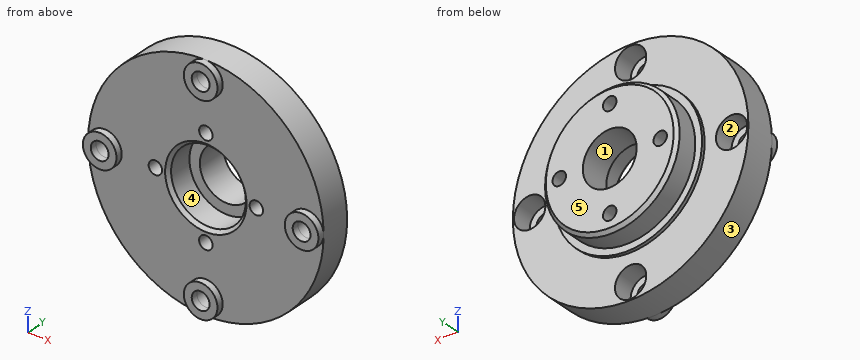
```python
from build123d import *

# Parameters (mm, degrees)
SKETCH1_R           = 35
SKETCH1_R_2         = 11.1
SKETCH1_R_3         = 2.65
BOSS_EXTRUDE1_DEPTH = 3
SKETCH2_R           = 35
SKETCH2_R_2         = 4.65
SKETCH2_R_3         = 11.1
BOSS_EXTRUDE2_DEPTH = 6
SKETCH3_R           = 11.1
SKETCH3_R_2         = 8
BOSS_EXTRUDE3_DEPTH = 1
SKETCH4_R           = 20
SKETCH4_R_2         = 8
BOSS_EXTRUDE4_DEPTH = 8
SKETCH5_R           = 22
SKETCH5_R_2         = 20
BOSS_EXTRUDE5_DEPTH = 1
SKETCH6_R           = 5
SKETCH6_R_2         = 2.65
BOSS_EXTRUDE6_DEPTH = 2
SKETCH7_R           = 2
CUT_EXTRUDE1_DEPTH  = 20
CHAMFER1_SIZE       = 1


with BuildPart() as part:
    # Sketch1 → Boss-Extrude1 (new body)
    with BuildSketch(Plane(origin=(0, 0, 0), x_dir=(1, 0, 0), z_dir=(0, 1, 0))):
        Circle(SKETCH1_R)
        Circle(SKETCH1_R_2, mode=Mode.SUBTRACT)
        with Locations((0, 30)):
            Circle(SKETCH1_R_3, mode=Mode.SUBTRACT)
        with Locations((30, 0)):
            Circle(SKETCH1_R_3, mode=Mode.SUBTRACT)
        with Locations((0, -30)):
            Circle(SKETCH1_R_3, mode=Mode.SUBTRACT)
        with Locations((-30, 0)):
            Circle(SKETCH1_R_3, mode=Mode.SUBTRACT)
    extrude(amount=BOSS_EXTRUDE1_DEPTH)

    # Sketch2 → Boss-Extrude2 (add)
    with BuildSketch(Plane(origin=(0, 3, 0), x_dir=(1, 0, 0), z_dir=(0, 1, 0))):
        Circle(SKETCH2_R)
        with Locations((0, -30)):
            Circle(SKETCH2_R_2, mode=Mode.SUBTRACT)
        with Locations((30, 0)):
            Circle(SKETCH2_R_2, mode=Mode.SUBTRACT)
        with Locations((0, 30)):
            Circle(SKETCH2_R_2, mode=Mode.SUBTRACT)
        with Locations((-30, 0)):
            Circle(SKETCH2_R_2, mode=Mode.SUBTRACT)
        Circle(SKETCH2_R_3, mode=Mode.SUBTRACT)
    extrude(amount=BOSS_EXTRUDE2_DEPTH)

    # Sketch3 → Boss-Extrude3 (add)
    with BuildSketch(Plane(origin=(0, 9, 0), x_dir=(1, 0, 0), z_dir=(0, 1, 0))):
        Circle(SKETCH3_R)
        Circle(SKETCH3_R_2, mode=Mode.SUBTRACT)
    extrude(amount=-BOSS_EXTRUDE3_DEPTH)

    # Sketch4 → Boss-Extrude4 (add)
    with BuildSketch(Plane(origin=(0, 9, 0), x_dir=(1, 0, 0), z_dir=(0, 1, 0))):
        Circle(SKETCH4_R)
        Circle(SKETCH4_R_2, mode=Mode.SUBTRACT)
    extrude(amount=BOSS_EXTRUDE4_DEPTH)

    # Sketch5 → Boss-Extrude5 (add)
    with BuildSketch(Plane(origin=(0, 9, 0), x_dir=(1, 0, 0), z_dir=(0, 1, 0))):
        Circle(SKETCH5_R)
        Circle(SKETCH5_R_2, mode=Mode.SUBTRACT)
    extrude(amount=BOSS_EXTRUDE5_DEPTH)

    # Sketch6 → Boss-Extrude6 (add)
    with BuildSketch(Plane(origin=(0, 0, 0), x_dir=(-1, 0, 0), z_dir=(0, -1, 0))):
        with Locations((30, 0)):
            Circle(SKETCH6_R)
        with Locations((30, 0)):
            Circle(SKETCH6_R_2, mode=Mode.SUBTRACT)
        with Locations((0, -30)):
            Circle(SKETCH6_R)
        with Locations((0, -30)):
            Circle(SKETCH6_R_2, mode=Mode.SUBTRACT)
        with Locations((-30, 0)):
            Circle(SKETCH6_R)
        with Locations((-30, 0)):
            Circle(SKETCH6_R_2, mode=Mode.SUBTRACT)
        with Locations((0, 30)):
            Circle(SKETCH6_R)
        with Locations((0, 30)):
            Circle(SKETCH6_R_2, mode=Mode.SUBTRACT)
    extrude(amount=BOSS_EXTRUDE6_DEPTH)

    # Sketch7 → Cut-Extrude1 (cut, through all)
    with BuildSketch(Plane(origin=(0, 17, 0), x_dir=(1, 0, 0), z_dir=(0, 1, 0))):
        with Locations((0, 15)):
            Circle(SKETCH7_R)
        with Locations((15, 0)):
            Circle(SKETCH7_R)
        with Locations((0, -15)):
            Circle(SKETCH7_R)
        with Locations((-15, 0)):
            Circle(SKETCH7_R)
    extrude(amount=-CUT_EXTRUDE1_DEPTH, mode=Mode.SUBTRACT)

    # Chamfer1
    chamfer1_edges = [part.edges().sort_by_distance(p)[0] for p in [
        (-11.1, 0, 0),
        (-20, 17, 0),
    ]]
    chamfer(chamfer1_edges, length=CHAMFER1_SIZE)


solid = part.part
```
Model file for the job. Use its own axes, mm. Face numbers are marked on the shaded views. A direction names the side the tool comes from. Coordinates: 2 decimals unless noted, no trailing zeros. Order: outer loops, then holes, each group sorted by start corner. A loop starts at its lowest first (then second) coordinate and runs counter-clockwise, first axis right, second up. Notation, with made-up numbers: (19, 77.5) -> (51, 77.5) arc R20 cw to (51, 104.5) -> close; hole circle Ø9 at (43, 13). An arc over 180 degrees is marked (long way). Answer as a JSON object with one key per item and string values. Group by question number.
1) Cut at C-C, the plane x = -30. Write the cut outline in (y, z), then the cut area to 3 significant figures.
2) Which spindle directions (+Z, -Z, +X, -X, +Y, -Y) get a long thin tool onto all of the face, cutting with end or side? Do the marked faces 1 and 2. Say none if no direction does.
3) Cut at A-A, the plane y = 12.25. Write the cut outline in (x, z).
4) Flat gauge pins, fed straight in: pin 1 (6 mm diameter, centred on x = 0, z = 30, fed in from +Y); pin 2 (5 mm diameter, centred on y = 3.5, z = -12.5, fed in from +X); pin 3 (2 mm diameter, centred on x = -15.5, y = 14, fed in from -Z) (3 decimals); pin 4 (6.5 mm diameter, centred on x = -3.5, z = 0, fed in from -Y). Where does each tip first touch, or does it go through?
5) Pull direction Z, two halves, no side cores. Call the marked faces 3, 4 and 5: +Z half, -Z half, draft (parallel to the pull), parting line (faces both ways), or undercut.
6) Drill centre lines: L1, parallel to X at y = 3.75, z = 0; L2, parallel to X at y = -0.25, z = -1.5. Where is each one in solid material? Low to high.
7) Cut at B-B, the plane z = -30. Write the cut outline in (x, y).
8) Cut at D-D, the plane z = -1. Count the separate pieces of the cut face and the enclosed holes in it, then the cut area to 3 significant figures.
Check values:
{
 "1": {"outline": "(-2, -5) -> (0, -5) -> (0, -18.03) -> (9, -18.03) -> (9, -4.65) -> (3, -4.65) -> (3, -2.65) -> (-2, -2.65) -> close; (-2, 2.65) -> (3, 2.65) -> (3, 4.65) -> (9, 4.65) -> (9, 18.03) -> (0, 18.03) -> (0, 5) -> (-2, 5) -> close", "area": "262 mm²"},
 "2": {"face 1": "+Y, -Y", "face 2": "+Y"},
 "3": {"outline": "circle Ø40 at (0, 0); hole circle Ø4 at (-15, 0); hole circle Ø16 at (0, 0); hole circle Ø4 at (0, -15); hole circle Ø4 at (0, 15); hole circle Ø4 at (15, 0)"},
 "4": {"pin 1": "stops at y = 3", "pin 2": "stops at x = 33.54", "pin 3": "stops at z = -13.775", "pin 4": "passes through"},
 "5": {"face 3": "parting line", "face 4": "undercut", "face 5": "draft"},
 "6": {"L1": "x = -35 to -34.65, -25.35 to -17, -13 to -11.1, 11.1 to 13, 17 to 25.35, 34.65 to 35", "L2": "x = -34.77 to -32.18, -27.82 to -25.23, 25.23 to 27.82, 32.18 to 34.77"},
 "7": {"outline": "(-18.03, 0) -> (-5, 0) -> (-5, -2) -> (-2.65, -2) -> (-2.65, 3) -> (-4.65, 3) -> (-4.65, 9) -> (-18.03, 9) -> close; (2.65, -2) -> (5, -2) -> (5, 0) -> (18.03, 0) -> (18.03, 9) -> (4.65, 9) -> (4.65, 3) -> (2.65, 3) -> close"},
 "8": {"separate pieces": "6", "enclosed holes": "0", "area": "395 mm²"}
}
